Autodesk Inventor part; units mm, degrees
ref_plane "YZ Plane" through (0, 0, 0) normal (1, 0, 0) x (0, 1, 0)
ref_plane "XZ Plane" through (0, 0, 0) normal (0, 1, 0) x (-1, 0, 0)
ref_plane "XY Plane" through (0, 0, 0) normal (0, 0, 1) x (1, 0, 0)
sketch "Sketch1" plane through (0, 0, 0) normal (0, 0, 1) x (1, 0, 0)
  line L0 (0, 0) -> (152.4, 0)
  line L1 (152.4, 0) -> (152.4, 152.4)
  line L2 (152.4, 152.4) -> (0, 152.4)
  line L3 (0, 152.4) -> (0, 0)
  line L4 (0, 3.175) -> (3.175, 0)
  circle A0 centre (15.24, 15.24) radius 1.143
  circle A1 centre (45.72, 15.24) radius 1.143
  circle A2 centre (76.2, 15.24) radius 1.143
  circle A3 centre (106.68, 15.24) radius 1.143
  circle A4 centre (137.16, 15.24) radius 1.143
  circle A5 centre (15.24, 45.72) radius 1.143
  circle A6 centre (45.72, 45.72) radius 1.143
  circle A7 centre (76.2, 45.72) radius 1.143
  circle A8 centre (106.68, 45.72) radius 1.143
  circle A9 centre (137.16, 45.72) radius 1.143
  circle A10 centre (15.24, 76.2) radius 1.143
  circle A11 centre (45.72, 76.2) radius 1.143
  circle A12 centre (76.2, 76.2) radius 1.143
  circle A13 centre (106.68, 76.2) radius 1.143
  circle A14 centre (137.16, 76.2) radius 1.143
  circle A15 centre (15.24, 106.68) radius 1.143
  circle A16 centre (45.72, 106.68) radius 1.143
  circle A17 centre (76.2, 106.68) radius 1.143
  circle A18 centre (106.68, 106.68) radius 1.143
  circle A19 centre (137.16, 106.68) radius 1.143
  circle A20 centre (15.24, 137.16) radius 1.143
  circle A21 centre (45.72, 137.16) radius 1.143
  circle A22 centre (76.2, 137.16) radius 1.143
  circle A23 centre (106.68, 137.16) radius 1.143
  circle A24 centre (137.16, 137.16) radius 1.143
  circle A25 centre (91.44, 60.96) radius 3.175
  dimension "d0" = 152.4
  dimension "d1" = 152.4
  dimension "d2" = 3.175
  dimension "d3" = 3.175
  dimension "d4" = 2.286
  dimension "d5" = 15.24
  dimension "d6" = 15.24
  dimension "d9" = 30.48
  dimension "d12" = 30.48
  dimension "d15" = 91.44
  dimension "d16" = 60.96
  dimension "d17" = 6.35
extrude "Extrusion1" add sketch "Sketch1" against normal blind 1.5 contours L4 L3 L2 L1 L0
equation "\"d3\" = d2"
properties part number "PCB RGB"
Verification items for the finished model (mm, model axes). Coordinates: 2 decimals unless noted, no trailing zeros. Loops run counter-clockwise (first coordinate to the right, second up) from the corner with the lowest first, then second, coordinate; pieces in that order, holes last. Notation, with made-up numbers: (64, 42) -> (98, 42) arc R20 ccw to (98, 49) -> close; hole circle Ø7 at (-7.75, 81.5). An arc over 180 degrees is marked (long way). Answer in a Markdown table with one row per item. Add a question column.
1. Section check B-B, the plane y = 60.96. Enter the section's corners in (x, z) (3 decimals), then the cut area to 3 significant figures.
2. Section check A-A, the plane x = 91.44. Enter the section's corners in (y, z) (3 decimals).
3. Material ranges on probe 1 along Y at (x, z) = (76.2, -0.6); probe 2 along X at (y, z) = (15.5, -0.1), recorded low to high. Write a range as [from, to].
4. Draft check along Y on faces 1 (the face through (75, 77, 0)), 2 (the face through (88.27, 61.1, -0.74)). Enter one of: +Y half, -Y half, draft (parallel to the pull), parting line (faces both ways), or undercut.
Derived:
| question | item | result |
|---|---|---|
| 1 | outline | (0, -1.5) -> (88.265, -1.5) -> (88.265, 0) -> (0, 0) -> close; (94.615, -1.5) -> (152.4, -1.5) -> (152.4, 0) -> (94.615, 0) -> close |
| 1 | area | 219 mm² |
| 2 | outline | (0, -1.5) -> (57.785, -1.5) -> (57.785, 0) -> (0, 0) -> close; (64.135, -1.5) -> (152.4, -1.5) -> (152.4, 0) -> (64.135, 0) -> close |
| 3 | probe 1 | y = [0, 14.1], [16.38, 44.58], [46.86, 75.06], [77.34, 105.54], [107.82, 136.02], [138.3, 152.4] |
| 3 | probe 2 | x = [0, 14.13], [16.35, 44.61], [46.83, 75.09], [77.31, 105.57], [107.79, 136.05], [138.27, 152.4] |
| 4 | face 1 | draft |
| 4 | face 2 | undercut |
